Read the model definition and answer for the solid it produces. Units are mm, in the model's axes. Face numbers are marked on the shaded views. A direction names the side the tool comes from. Coordinates: 2 decimals unless noted, no trailing zeros. Write each loop counter-clockwise with the first axis right and the second up, starting at its lowest first coordinate (ties: lowest second). Pieces come first, ordered by that corner, then holes.
(1) The part is cut by section B-B, the plane z = 1.9. Determine the outline of the cut face in (x, y) (3 decimals), and give its area (3 significant figures).
(2) Which of the six approach directions +Z, -Z, +X, -X, +Y, -Y give full straight-line access (tool end or side, diameter ignored) to the marked faces 1, 2 and 3?
(3) The part is cut by section A-A, the plane y = -4.5. Determine the outline of the cut face in (x, z) (3 decimals), and give its area (3 significant figures).
(4) Straight lines are drawn through the part: line 1 along X through (y, z) = (-1.25, 1.1) (3 decimals); line 2 along X through (y, z) = (1.5, 0.35) (3 decimals); line 3 along Y through (x, z) = (-6, 2.85) (3 decimals). For each, find the intervals that lie inside material, in ascending order.
(5) The part is cut by section C-C, the plane x = 1. Determine the outline of the cut face in (y, z) (3 decimals).
(6) Determine the mould class of the marked faces 4, 5 and 6 for opening direction X: pulls with the +X half, pulls with the -X half, needs draft (parallel to the pull), parting line crosses it, or undercut.
Autodesk Fusion 360 part; units mm, degrees
sketch "Sketch1" plane through (0, 0, 0) normal (0, 0, 1) x (1, 0, 0)
  line L0 (0, 18.1881) -> (0, -15.507) construction
  line L1 (-13.7826, 0) -> (15.7817, 0) construction
  line L2 (6.295, 6.295) -> (-6.295, 6.295) construction
  line L3 (-6.295, 6.295) -> (-6.295, -6.295)
  line L4 (-6.295, -6.295) -> (6.295, -6.295) construction
  line L5 (6.295, -6.295) -> (6.295, 6.295)
  line L6 (6.295, 6.295) -> (-6.295, -6.295) construction
  line L7 (-6.295, 6.295) -> (6.295, -6.295) construction
  line L8 (-6.295, 6.295) -> (0, 6.575)
  line L9 (6.295, 6.295) -> (0, 6.575)
  line L10 (6.295, -6.295) -> (0, -6.575)
  line L11 (-6.295, -6.295) -> (0, -6.575)
  arc A0 (-5.8172, 6.3163) -> (-6.295, 5.8167) centre (-5.795, 5.8167) ccw
  arc A1 (-6.295, -5.8167) -> (-5.8172, -6.3163) centre (-5.795, -5.8167) ccw
  arc A2 (5.8172, -6.3163) -> (6.295, -5.8167) centre (5.795, -5.8167) ccw
  arc A3 (6.295, 5.8167) -> (5.8172, 6.3163) centre (5.795, 5.8167) ccw
  line L12 (-7.695, 7.695) -> (-7.695, -7.695)
  line L13 (-7.695, -7.695) -> (7.695, -7.695)
  line L14 (7.695, -7.695) -> (7.695, 7.695)
  line L15 (7.695, 7.695) -> (-7.695, 7.695)
  dimension "d8" = 12.59
  dimension "d9" = 12.59
  dimension "d10" = 0.28
  dimension "d11" = 0.5
  dimension "d12" = 0.5
  dimension "d13" = 1.4
extrude "Extrude1" add sketch "Sketch1" along normal blind 3 contours L3 L8 A0 | L3 L11 A1 | L5 L9 A3 | L5 L10 A2 | L12 L13 L14 L15
sketch "Sketch3" plane through (0, 0, 0) normal (0, 1, 0) x (1, 0, 0)
  line L0 (6.295, 0) -> (6.295, -3)
  line L1 (6.295, -3) -> (6.295, 0)
  line L2 (-6.295, 0) -> (-6.295, -3)
  line L3 (-6.295, -3) -> (-6.295, 0)
  arc A0 (6.295, 0) -> (6.295, -0.8) centre (6.7422, -0.4) ccw
  line L4 (0, -4.7856) -> (0, 3.5594) construction
  arc A1 (-6.295, -0.8) -> (-6.295, 0) centre (-6.7422, -0.4) ccw
  dimension "d16" = 0.8
  dimension "d17" = 0.6
extrude "Extrude2" add sketch "Sketch3" along normal mid plane 8
fillet "Fillet2" radius 1 4 edges at (7.695, -7.695, 1.5) (7.695, 7.695, 1.5) (-7.695, 7.695, 1.5) (-7.695, -7.695, 1.5)
chamfer "Chamfer1" distance 0.3 angle 45 12 edges at (2.9086, 6.4456, 0) (6.1563, 6.1624, 0) (6.295, 4.9084, 0) (-2.9086, 6.4456, 0) (-6.295, 4.9084, 0) (-6.1563, 6.1624, 0) (-2.9086, -6.4456, 0) (-6.1563, -6.1624, 0) (-6.295, -4.9084, 0) (2.9086, -6.4456, 0) (6.295, -4.9084, 0) (6.1563, -6.1624, 0)
chamfer "Chamfer2" distance 0.3 angle 45 1 faces at (7.2283, 1.9389, 3)
equation "d9 = d8"
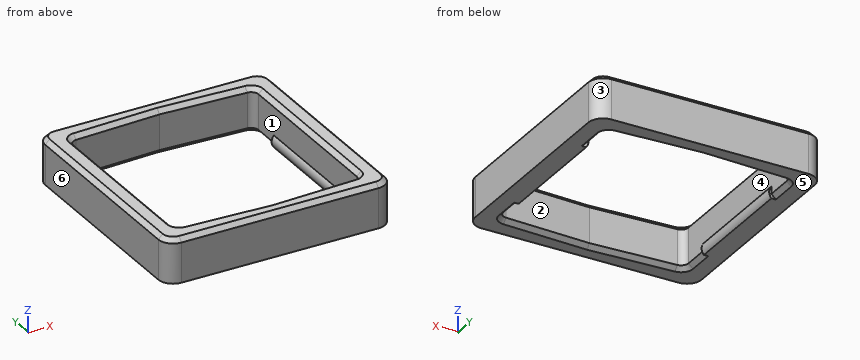
Computed:
1. outline: (-7.695, -6.695) arc R1 ccw to (-6.695, -7.695) - (6.695, -7.695) arc R1 ccw to (7.695, -6.695) - (7.695, 6.695) arc R1 ccw to (6.695, 7.695) - (-6.695, 7.695) arc R1 ccw to (-7.695, 6.695) - close; hole (-6.295, -5.817) arc R0.5 ccw to (-5.817, -6.316) - (0, -6.575) - (5.817, -6.316) arc R0.5 ccw to (6.295, -5.817) - (6.295, 5.817) arc R0.5 ccw to (5.817, 6.316) - (0, 6.575) - (-5.817, 6.316) arc R0.5 ccw to (-6.295, 5.817) - close
1. area: 74.2 mm2
2. face 1: +Z
2. face 2: +Z, -Z
2. face 3: +Z, -Z, +X, +Y
3. outline: (-7.695, 0) - (-6.595, 0) - (-6.295, 0.3) - (-6.295, 2.7) - (-6.595, 3) - (-7.395, 3) - (-7.695, 2.7) - close; (6.295, 0.3) - (6.595, 0) - (7.695, 0) - (7.695, 2.7) - (7.395, 3) - (6.595, 3) - (6.295, 2.7) - close
3. area: 8.13 mm2
4. line 1: x = -7.695 to -6.295, 6.295 to 7.695
4. line 2: x = -7.695 to -6.144, 6.144 to 7.695
4. line 3: y = -7.545 to -6.434, 6.434 to 7.545
5. outline: (-7.695, 0) - (-6.831, 0) - (-6.531, 0.3) - (-6.531, 2.7) - (-6.831, 3) - (-7.395, 3) - (-7.695, 2.7) - close; (6.531, 0.3) - (6.831, 0) - (7.695, 0) - (7.695, 2.7) - (7.395, 3) - (6.831, 3) - (6.531, 2.7) - close
6. face 4: undercut
6. face 5: needs draft
6. face 6: pulls with the -X half
